Geometry: final body of the model. Coordinates: model frame, mm. Face numbers are marked on the shaded views. A direction names the side the tool comes from. Round coordinates to 2 decimals unless told otherwise and drop trailing zeros. Loops run counter-clockwise (first coordinate to the right, second up) from the corner with the lowest first, then second, coordinate; pieces in that order, holes last. Notation, with made-up numbers: M -12,22.25 L 14,22.25 A24 ccw 14,49.25 Z; hole C 46.5,5.5 d10. An arc over 180 degrees is marked long. Write each question's results on one line, items separated by ' | '.
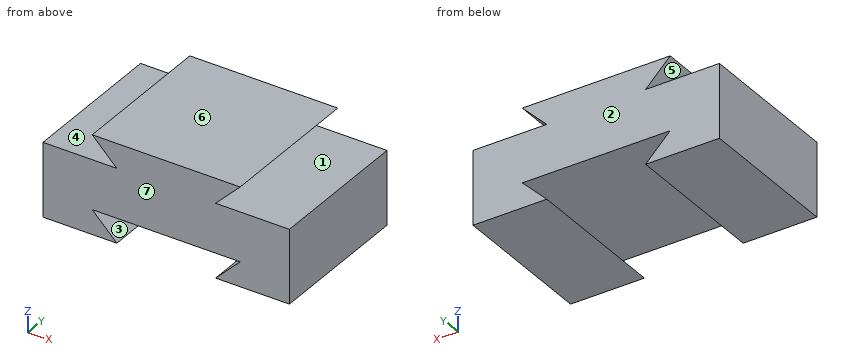
```python
from build123d import *

# Parameters (mm, degrees)
F0_W     = 38.1
F0_H     = 76.2
F1_DEPTH = 12.7
F2_SIZE  = 12.69999
F3_W     = 76.2
F3_H     = 76.2
F4_DEPTH = 25.4
F5_W     = 50.8
F5_H     = 76.2
F6_DEPTH = 12.7
F8_DEPTH = 76.201


# Not quite as in the source:
# - a fillet or chamfer is up to 0.001 mm smaller than in the source, because OpenCascade refuses the exact size


with BuildPart() as f1:
    # F0 (on Top) → F1 (new body)
    with BuildSketch(Plane.XY):
        with Locations((-44.5209794172, 0.8258419111)):
            Rectangle(F0_W, F0_H)
    extrude(amount=F1_DEPTH)

    # F2 (size 12.7 in the source; OpenCascade refuses exactly that, so slightly less here)
    f2_edges = [f1.edges().sort_by_distance(p)[0] for p in [
        (-25.470979, 0.825842, 12.7),
    ]]
    chamfer(f2_edges, length=F2_SIZE)

    # F3 (on face) → F4 (join)
    with BuildSketch(Plane.XY.offset(12.7)):
        with Locations((-25.4709794172, 0.8258419111)):
            Rectangle(F3_W, F3_H)
    extrude(amount=F4_DEPTH)

    # F5 (on face) → F6 (join)
    with BuildSketch(Plane.XY.offset(38.1)):
        with Locations((-12.7709794172, 0.8258419111)):
            Rectangle(F5_W, F5_H)
    extrude(amount=F6_DEPTH)

    # F7 (on face) → F8 (cut, through all)
    with BuildSketch(Plane.XZ.offset(37.2741580889)):
        Polygon((-38.1709794172, 50.8), (-38.1709794172, 38.1), (-25.4709794172, 38.1), align=None)
    extrude(amount=-F8_DEPTH, mode=Mode.SUBTRACT)

    # F9: F1 across plane


with BuildPart() as f1_1:
    add(f1.part)
    add(f1.part.mirror(Plane.YZ))


solid = f1_1.part
```
1. Section C-C (x = -33.5). Output: boundary loops of the cut face in (y, z).
Answer key:
outline: M -37.27,0 L 38.93,0 L 38.93,8.03 L -37.27,8.03 Z; M -37.27,12.7 L 38.93,12.7 L 38.93,38.1 L -37.27,38.1 Z; M -37.27,46.13 L 38.93,46.13 L 38.93,50.8 L -37.27,50.8 Z
2. Ray query, probe 1 along Z at (x, y) = (27, 23.5); probe 2 along Z at (x, y) = (-32, -32); probe 3 along Z at (x, y) = (-16, 28). Return the intervals inside material, ascending.
Answer key:
probe 1: z = 0 to 1.53, 12.7 to 38.1, 39.63 to 50.8 | probe 2: z = 0 to 6.53, 12.7 to 38.1, 44.63 to 50.8 | probe 3: z = 12.7 to 50.8
3. Draft query along Z for the marked faces 4, 5, 6 and 7. Return one class per face: pulls with the +Z half, pulls with the -Z half, needs draft (parallel to the pull), parting line crosses it, or undercut.
Answer key:
face 4: undercut | face 5: undercut | face 6: pulls with the +Z half | face 7: needs draft
4. Access query for the marked faces 1, 2 and 3. Directions: +Z, -Z, +X, -X, +Y, -Y. A direction counts if a zero-diameter tool reaches every point of the face in a straight line with its end or side. Return the directions, or none.
Answer key:
face 1: +X, +Y, -Y | face 2: +Z, -Z, +X, -X, +Y | face 3: +Y, -Y
5. Pin query (flat end, axial travel): P1, Ø11.5, axis at x = -49.5, y = 15, coming from the +Z side. Return the tip coordinate at first contact, or that it passes through.
Answer key:
P1: stops at z = 38.1
6. Section B-B (z = 8.5). Output: boundary loops of the cut face in (x, y).
Answer key:
outline: M -63.57,-37.27 L -33.97,-37.27 L -33.97,38.93 L -63.57,38.93 Z; M 33.97,-37.27 L 63.57,-37.27 L 63.57,38.93 L 33.97,38.93 Z
7. Section D-D (x = -12.5). Output: boundary loops of the cut face in (y, z), then the cut area to 3 significant figures.
Answer key:
outline: M -37.27,12.7 L 38.93,12.7 L 38.93,50.8 L -37.27,50.8 Z | area: 2,900 mm²
